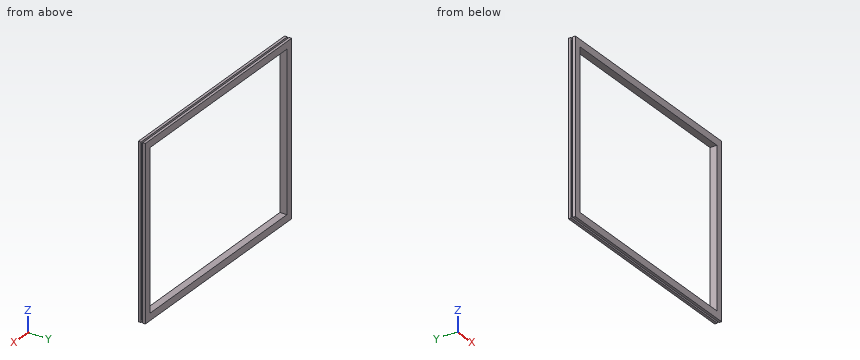
```python
from build123d import *

# Parameters (mm, degrees)
SKETCH1_W               = 1250
SKETCH1_H               = 970
SKETCH1_W_2             = 1170
SKETCH1_H_2             = 890
BOSS_EXTRUDE1_DEPTH     = 40
CUT_EXTRUDE1_DEPTH      = 1155.610323876
CUT_EXTRUDE1_DEPTH_BACK = 1155.610323876
SKETCH2_W               = 10
SKETCH2_H               = 10
CUT_EXTRUDE2_DEPTH      = 1342.389205264
CUT_EXTRUDE2_DEPTH_BACK = 1342.389205264
SKETCH3_W               = 10
SKETCH3_H               = 10


with BuildPart() as part:
    # Sketch1 → Boss-Extrude1 (new body)
    with BuildSketch(Plane(origin=(0, 0, 0), x_dir=(1, 0, 0), z_dir=(0, 1, 0))):
        Rectangle(SKETCH1_W, SKETCH1_H)
        Rectangle(SKETCH1_W_2, SKETCH1_H_2, mode=Mode.SUBTRACT)
    extrude(amount=BOSS_EXTRUDE1_DEPTH)

    # Sketch2 → Cut-Extrude1 (cut, two sides: drawn at the far end of the back side and taken through both)
    with BuildSketch(Plane.XY.offset(485).offset(-CUT_EXTRUDE1_DEPTH_BACK)):
        with Locations((-620, 20)):
            Rectangle(SKETCH2_W, SKETCH2_H)
        with Locations((620, 20)):
            Rectangle(SKETCH2_W, SKETCH2_H)
    extrude(amount=CUT_EXTRUDE1_DEPTH + CUT_EXTRUDE1_DEPTH_BACK, mode=Mode.SUBTRACT)

    # Sketch3 → Cut-Extrude2 (cut, two sides: drawn at the far end of the back side and taken through both)
    with BuildSketch(Plane.ZY.offset(625).offset(-CUT_EXTRUDE2_DEPTH_BACK)):
        with Locations((480, 20)):
            Rectangle(SKETCH3_W, SKETCH3_H)
        with Locations((-480, 20)):
            Rectangle(SKETCH3_W, SKETCH3_H)
    extrude(amount=CUT_EXTRUDE2_DEPTH + CUT_EXTRUDE2_DEPTH_BACK, mode=Mode.SUBTRACT)


solid = part.part
```
Check sheet for the modelled part. Datum: model origin and axes. Units: mm. Round coordinates to 2 decimals unless told otherwise and drop trailing zeros. Order: outer loops, then holes, each group sorted by start corner. A loop starts at its lowest first (then second) coordinate and runs counter-clockwise, first axis right, second up.
1) Scan lines: line 1 (X direction, y = 6.5, z = 199.5); line 2 (Z direction, x = -66.5, y = 2.5); line 3 (Z direction, x = 514, y = 17). Record each from-to range of solid material in increasing order.
2) Section check C-C (y = 31.5). Record the boundary of the cut face in (x, z), and give its area (3 significant figures).
3) Section check B-B (x = -216). Record the boundary of the cut face in (y, z).
4) Section check A-A (z = 364). Record the boundary of the cut face in (x, y).
5) Go/stop test with flat-tipped pins: pin 1 Ø1 at (y, z) = (19.5, 90.5) entering from +X; pin 2 Ø8 at (x, y) = (-64, 19.5) entering from -Z; pin 3 Ø3 at (y, z) = (18, 194.5) entering from -X. Record where each tip stops, or that it passes through.
Result:
1. line 1: x = -625 to -585, 585 to 625
1. line 2: z = -485 to -445, 445 to 485
1. line 3: z = -475 to -445, 445 to 475
2. outline: (-625, -485) - (625, -485) - (625, 485) - (-625, 485) - close; hole (-585, -445) - (585, -445) - (585, 445) - (-585, 445) - close
2. area: 171,000 mm2
3. outline: (0, -485) - (15, -485) - (15, -475) - (25, -475) - (25, -485) - (40, -485) - (40, -445) - (0, -445) - close; (0, 445) - (40, 445) - (40, 485) - (25, 485) - (25, 475) - (15, 475) - (15, 485) - (0, 485) - close
4. outline: (-625, 0) - (-585, 0) - (-585, 40) - (-625, 40) - (-625, 25) - (-615, 25) - (-615, 15) - (-625, 15) - close; (585, 0) - (625, 0) - (625, 15) - (615, 15) - (615, 25) - (625, 25) - (625, 40) - (585, 40) - close
5. pin 1: stops at x = 615
5. pin 2: stops at z = -475
5. pin 3: stops at x = -615
